Autodesk Inventor part; units mm, degrees
ref_plane "YZ Plane" through (0, 0, 0) normal (1, 0, 0) x (0, 1, 0)
ref_plane "XZ Plane" through (0, 0, 0) normal (0, 1, 0) x (-1, 0, 0)
ref_plane "XY Plane" through (0, 0, 0) normal (0, 0, 1) x (1, 0, 0)
sketch "Skizze1" plane through (0, 0, 0) normal (0, 0, 1) x (1, 0, 0)
  circle A0 centre (0, 0) radius 30
  dimension "d0" = 60
extrude "Extrusion1" add sketch "Skizze1" along normal blind 4
sketch "Skizze2" plane through (0, 0, 4) normal (0, 0, 1) x (1, 0, 0)
  line L0 (14, 17.5) -> (20, 17.5)
  line L1 (20, -17.5) -> (14, -17.5)
  line L2 (20, 11.5) -> (14, 11.5)
  line L3 (20, -11.5) -> (14, -11.5)
  line L4 (-42, 0) -> (42, 0)
  line L5 (14, -17.5) -> (14, -11.5)
  line L6 (14, 11.5) -> (14, 17.5)
  line L7 (20, 17.5) -> (20, 11.5)
  line L8 (20, -11.5) -> (20, -17.5)
  point P0 (0, 0)
  point P1 (14, 0)
  dimension "d5" = 6
  dimension "d6" = 35
  dimension "d9" = 23
  dimension "d10" = 14
extrude "Extrusion2" add sketch "Skizze2" along normal blind 22
sketch "Skizze3" plane through (14, -17.5, 4) normal (-1, 0, 0) x (0, 0, 1)
  line L0 (22, 35) -> (22, 29)
  line L1 (22, 6) -> (22, 0)
  line L2 (0, 0) -> (22, 0)
  line L3 (-4, 17.5) -> (14.084, 17.5)
  line L4 (0, -12.5) -> (0, 47.5)
  point P0 (16, 4)
  point P1 (16, 31)
  point P2 (22, 3)
  point P3 (22, 32)
  dimension "d13" = 27
  dimension "d14" = 16
hole "Bohrung1" at (14, -13.5, 20) at (14, 13.5, 20) direction (1, 0, 0) diameter 1 depth 6.5 tip angle 118
fillet "Rundung2" radius 1 1 edges at (-30, 0, 4)
sketch "Skizze6" plane through (14, 11.5, 4) normal (-1, 0, 0) x (0, 0, 1)
  line L0 (0, -23) -> (22, -23)
  line L1 (0, 0) -> (22, 0)
  line L2 (0, 0) -> (10, 0)
  line L3 (10, 0) -> (10, -23)
  line L4 (10, -23) -> (0, -23)
  line L5 (0, -23) -> (0, 0)
  point P0 (-4, -11.5)
  point P1 (0.5, -23)
  point P2 (21.5, -23)
  point P3 (21.5, 0)
  point P4 (0.5, -23)
  point P5 (10, 0)
  dimension "d30" = 10
extrude "Extrusion4" add sketch "Skizze6" against normal up to surface (6 mm away)
chamfer "Fasen2" distance 0.4 angle 45 8 edges at (14, 11.5, 20) (17, 11.5, 26) (20, 11.5, 20) (14, 0, 14) (14, -11.5, 20) (17, -11.5, 26) (20, -11.5, 20) (20, 0, 14)
fillet "Rundung3" radius 0.4 14 edges at (14, 0, 4) (14, -17.5, 15) (20, -17.5, 15) (17, -17.5, 26) (20, -14.7, 26) (14, -14.7, 26) (14, 14.7, 26) (20, 14.7, 26) (17, 17.5, 26) (14, 17.5, 15) (17, -17.5, 4) (20, 17.5, 15) (20, 0, 4) (17, 17.5, 4)
properties part number "Shoulder"
Read the model definition and answer for the solid it produces. Units are mm, in the model's axes. A direction names the side the tool comes from. Coordinates: 2 decimals unless noted, no trailing zeros. Loops run counter-clockwise (first coordinate to the right, second up) from the corner with the lowest first, then second, coordinate; pieces in that order, holes last. Notation, with made-up numbers: (-36, 41) -> (10, 41) arc R27 cw to (10, 74) -> close; hole circle Ø1 at (-37.5, 67). An arc over 180 degrees is marked (long way). Write item = value, one per line. Start each with the question number.
1) The part is cut by section B-B, the plane x = 0. Determine the outline of the cut face in (y, z).
2) The part is cut by section C-C, the plane y = 0. Determine the outline of the cut face in (x, z), plus the area to 3 significant figures.
3) The part is cut by section D-D, the plane z = 12. Determine the outline of the cut face in (x, y), plus the area to 3 significant figures.
4) For faces 5 (the face through (17, 11.5, 20)), 6 (the face through (14, 0, 10)), 7 (the face through (0, 0, 0)), 8 (the face through (17, 17.5, 15)), 9 (the face through (20, 0, 10)), determine the directions among +Z, -Z, +X, -X, +Y, -Y from which every point of the face is accessible in a straight line to the end or side of a thin tool.
5) The mould has two halves that part along Y. Classify faces 1 (the face through (17, -11.5, 20)), 2 (the face through (17, -17.5, 15)), 3 (the face through (17, -14, 26)), 4 (the face through (-29.97, -1.32, 1.48)): pulls with the +Y half, pulls with the -Y half, needs draft (parallel to the pull), parting line crosses it, or undercut.
6) Find the intervals of material crossed by L1, parallel to Y at x = 16.25, z = 20; L2, parallel to Z at x = 18.8, y = 13.5; L3, parallel to X at y = 16, z = 9.5, in increasing order. Write a range as from..to.
7) Given P1, Ø10, axis at x = 5.5, z = 16, coming from the +Y side; P2, Ø4, axis at x = 17, y = 3.5, coming from the +Z side; P3, Ø6.5, axis at y = 2.5, z = 10, coming from the +X side; P4, Ø10, axis at x = -21, y = 3.5, coming from the +Z side, each flat-ended and moving along its own axis, determine where each tip first touches the part or whether it passes through.
8) The part is cut by section A-A, the plane z = 24. Determine the outline of the cut face in (x, y).
Result:
q1.outline = (-30, 0) -> (30, 0) -> (30, 3) arc R1 ccw to (29, 4) -> (-29, 4) arc R1 ccw to (-30, 3) -> close
q2.outline = (-30, 0) -> (30, 0) -> (30, 3) arc R1 ccw to (29, 4) -> (20.4, 4) arc R0.4 cw to (20, 4.4) -> (20, 13.6) -> (19.6, 14) -> (14.4, 14) -> (14, 13.6) -> (14, 4.4) arc R0.4 cw to (13.6, 4) -> (-29, 4) arc R1 ccw to (-30, 3) -> close
q2.area = 299 mm²
q3.outline = (14, -17.1) arc R0.4 ccw to (14.4, -17.5) -> (19.6, -17.5) arc R0.4 ccw to (20, -17.1) -> (20, 17.1) arc R0.4 ccw to (19.6, 17.5) -> (14.4, 17.5) arc R0.4 ccw to (14, 17.1) -> close
q3.area = 210 mm²
q4.face_5 = +Z, +X, -X
q4.face_6 = +Z, -X, +Y, -Y
q4.face_7 = -Z, +X, -X, +Y, -Y
q4.face_8 = +Z, +X, -X, +Y
q4.face_9 = +Z, +X, +Y, -Y
q5.face_1 = undercut
q5.face_2 = pulls with the -Y half
q5.face_3 = needs draft
q5.face_4 = parting line crosses it
q6.L1 = -17.5..-14, -13..-11.5, 11.5..13, 14..17.5
q6.L2 = 0..19.5, 20.5..26
q6.L3 = 14..20
q7.P1 = through
q7.P2 = 14
q7.P3 = 20
q7.P4 = 4
q8.outline = (14, -17.1) arc R0.4 ccw to (14.4, -17.5) -> (19.6, -17.5) arc R0.4 ccw to (20, -17.1) -> (20, -11.9) -> (19.6, -11.5) -> (14.4, -11.5) -> (14, -11.9) -> close; (14, 11.9) -> (14.4, 11.5) -> (19.6, 11.5) -> (20, 11.9) -> (20, 17.1) arc R0.4 ccw to (19.6, 17.5) -> (14.4, 17.5) arc R0.4 ccw to (14, 17.1) -> close
